from build123d import *

# Parameters (mm, degrees)
F0_R     = 9.75
F0_R_2   = 2.15
F1_DEPTH = 100


with BuildPart() as f1:
    # F0 (on Front) → F1 (new body)
    with BuildSketch(Plane.XZ):
        with Locations((6, 0)):
            Circle(F0_R)
        with Locations((3, -5.2)):
            Circle(F0_R_2, mode=Mode.SUBTRACT)
        with BuildLine():
            ThreePointArc((0.394847, -3.024334), (0.593975, -3.122706), (0.579462, -3.344334))
            ThreePointArc((0.579462, -3.344334), (-0.023044, -4.795398), (0.176673, -6.353832))
            ThreePointArc((0.176673, -6.353832), (0.105059, -6.594152), (-0.145019, -6.575618))
            ThreePointArc((-0.145019, -6.575618), (-1.795123, -4.498451), (-2.767969, -2.030449))
            ThreePointArc((-2.767969, -2.030449), (-2.65874, -1.804579), (-2.414779, -1.863154))
            ThreePointArc((-2.414779, -1.863154), (-1.164953, -2.818756), (0.394847, -3.024334))
        make_face(mode=Mode.SUBTRACT)
        with BuildLine():
            ThreePointArc((6.394847, -3.024334), (6.593975, -3.122706), (6.579462, -3.344334))
            ThreePointArc((6.579462, -3.344334), (6.359886, -3.672814), (6.184615, -4.026923))
            ThreePointArc((6.184615, -4.026923), (6, -4.15), (5.815385, -4.026923))
            ThreePointArc((5.815385, -4.026923), (5.640114, -3.672814), (5.420538, -3.344334))
            ThreePointArc((5.420538, -3.344334), (5.406025, -3.122706), (5.605153, -3.024334))
            ThreePointArc((5.605153, -3.024334), (6, -3.05), (6.394847, -3.024334))
        make_face(mode=Mode.SUBTRACT)
        with BuildLine():
            ThreePointArc((2.815385, -1.173077), (3, -1.05), (3.184615, -1.173077))
            ThreePointArc((3.184615, -1.173077), (3.359886, -1.527186), (3.579462, -1.855666))
            ThreePointArc((3.579462, -1.855666), (3.593975, -2.077294), (3.394847, -2.175666))
            ThreePointArc((3.394847, -2.175666), (3, -2.15), (2.605153, -2.175666))
            ThreePointArc((2.605153, -2.175666), (2.406025, -2.077294), (2.420538, -1.855666))
            ThreePointArc((2.420538, -1.855666), (2.640114, -1.527186), (2.815385, -1.173077))
        make_face(mode=Mode.SUBTRACT)
        with BuildLine():
            ThreePointArc((5.815385, -6.373077), (6, -6.25), (6.184615, -6.373077))
            ThreePointArc((6.184615, -6.373077), (7.139308, -7.616677), (8.585647, -8.221723))
            ThreePointArc((8.585647, -8.221723), (8.757847, -8.404014), (8.616624, -8.61123))
            ThreePointArc((8.616624, -8.61123), (6, -9), (3.383376, -8.61123))
            ThreePointArc((3.383376, -8.61123), (3.242153, -8.404014), (3.414353, -8.221723))
            ThreePointArc((3.414353, -8.221723), (4.860692, -7.616677), (5.815385, -6.373077))
        make_face(mode=Mode.SUBTRACT)
        with Locations((9, -5.2)):
            Circle(F0_R_2, mode=Mode.SUBTRACT)
        with BuildLine():
            ThreePointArc((8.815385, -1.173077), (9, -1.05), (9.184615, -1.173077))
            ThreePointArc((9.184615, -1.173077), (9.359886, -1.527186), (9.579462, -1.855666))
            ThreePointArc((9.579462, -1.855666), (9.593975, -2.077294), (9.394847, -2.175666))
            ThreePointArc((9.394847, -2.175666), (9, -2.15), (8.605153, -2.175666))
            ThreePointArc((8.605153, -2.175666), (8.406025, -2.077294), (8.420538, -1.855666))
            ThreePointArc((8.420538, -1.855666), (8.640114, -1.527186), (8.815385, -1.173077))
        make_face(mode=Mode.SUBTRACT)
        with BuildLine():
            ThreePointArc((11.420538, -3.344334), (11.406025, -3.122706), (11.605153, -3.024334))
            ThreePointArc((11.605153, -3.024334), (13.164953, -2.818756), (14.414779, -1.863154))
            ThreePointArc((14.414779, -1.863154), (14.65874, -1.804579), (14.767969, -2.030449))
            ThreePointArc((14.767969, -2.030449), (13.795123, -4.498451), (12.145019, -6.575618))
            ThreePointArc((12.145019, -6.575618), (11.894941, -6.594152), (11.823327, -6.353832))
            ThreePointArc((11.823327, -6.353832), (12.023044, -4.795398), (11.420538, -3.344334))
        make_face(mode=Mode.SUBTRACT)
        Circle(F0_R_2, mode=Mode.SUBTRACT)
        with BuildLine():
            ThreePointArc((0.579462, 3.344334), (0.593975, 3.122706), (0.394847, 3.024334))
            ThreePointArc((0.394847, 3.024334), (-1.164953, 2.818756), (-2.414779, 1.863154))
            ThreePointArc((-2.414779, 1.863154), (-2.65874, 1.804579), (-2.767969, 2.030449))
            ThreePointArc((-2.767969, 2.030449), (-1.795123, 4.498451), (-0.145019, 6.575618))
            ThreePointArc((-0.145019, 6.575618), (0.105059, 6.594152), (0.176673, 6.353832))
            ThreePointArc((0.176673, 6.353832), (-0.023044, 4.795398), (0.579462, 3.344334))
        make_face(mode=Mode.SUBTRACT)
        with BuildLine():
            ThreePointArc((3.184615, 1.173077), (3, 1.05), (2.815385, 1.173077))
            ThreePointArc((2.815385, 1.173077), (2.640114, 1.527186), (2.420538, 1.855666))
            ThreePointArc((2.420538, 1.855666), (2.406025, 2.077294), (2.605153, 2.175666))
            ThreePointArc((2.605153, 2.175666), (3, 2.15), (3.394847, 2.175666))
            ThreePointArc((3.394847, 2.175666), (3.593975, 2.077294), (3.579462, 1.855666))
            ThreePointArc((3.579462, 1.855666), (3.359886, 1.527186), (3.184615, 1.173077))
        make_face(mode=Mode.SUBTRACT)
        with Locations((3, 5.2)):
            Circle(F0_R_2, mode=Mode.SUBTRACT)
        with Locations((6, 0)):
            Circle(F0_R_2, mode=Mode.SUBTRACT)
        with BuildLine():
            ThreePointArc((9.184615, 1.173077), (9, 1.05), (8.815385, 1.173077))
            ThreePointArc((8.815385, 1.173077), (8.640114, 1.527186), (8.420538, 1.855666))
            ThreePointArc((8.420538, 1.855666), (8.406025, 2.077294), (8.605153, 2.175666))
            ThreePointArc((8.605153, 2.175666), (9, 2.15), (9.394847, 2.175666))
            ThreePointArc((9.394847, 2.175666), (9.593975, 2.077294), (9.579462, 1.855666))
            ThreePointArc((9.579462, 1.855666), (9.359886, 1.527186), (9.184615, 1.173077))
        make_face(mode=Mode.SUBTRACT)
        with BuildLine():
            ThreePointArc((5.605153, 3.024334), (5.406025, 3.122706), (5.420538, 3.344334))
            ThreePointArc((5.420538, 3.344334), (5.640114, 3.672814), (5.815385, 4.026923))
            ThreePointArc((5.815385, 4.026923), (6, 4.15), (6.184615, 4.026923))
            ThreePointArc((6.184615, 4.026923), (6.359886, 3.672814), (6.579462, 3.344334))
            ThreePointArc((6.579462, 3.344334), (6.593975, 3.122706), (6.394847, 3.024334))
            ThreePointArc((6.394847, 3.024334), (6, 3.05), (5.605153, 3.024334))
        make_face(mode=Mode.SUBTRACT)
        with Locations((12, 0)):
            Circle(F0_R_2, mode=Mode.SUBTRACT)
        with BuildLine():
            ThreePointArc((11.605153, 3.024334), (11.406025, 3.122706), (11.420538, 3.344334))
            ThreePointArc((11.420538, 3.344334), (12.023044, 4.795398), (11.823327, 6.353832))
            ThreePointArc((11.823327, 6.353832), (11.894941, 6.594152), (12.145019, 6.575618))
            ThreePointArc((12.145019, 6.575618), (13.795123, 4.498451), (14.767969, 2.030449))
            ThreePointArc((14.767969, 2.030449), (14.65874, 1.804579), (14.414779, 1.863154))
            ThreePointArc((14.414779, 1.863154), (13.164953, 2.818756), (11.605153, 3.024334))
        make_face(mode=Mode.SUBTRACT)
        with Locations((9, 5.2)):
            Circle(F0_R_2, mode=Mode.SUBTRACT)
        with BuildLine():
            ThreePointArc((6.184615, 6.373077), (6, 6.25), (5.815385, 6.373077))
            ThreePointArc((5.815385, 6.373077), (4.860692, 7.616677), (3.414353, 8.221723))
            ThreePointArc((3.414353, 8.221723), (3.242153, 8.404014), (3.383376, 8.61123))
            ThreePointArc((3.383376, 8.61123), (6, 9), (8.616624, 8.61123))
            ThreePointArc((8.616624, 8.61123), (8.757847, 8.404014), (8.585647, 8.221723))
            ThreePointArc((8.585647, 8.221723), (7.139308, 7.616677), (6.184615, 6.373077))
        make_face(mode=Mode.SUBTRACT)
    extrude(amount=F1_DEPTH)


solid = f1.part
Input: part model. Units: mm. Frame: model coordinates. Give positions to 0.01 mm unless a question says otherwise; leave off trailing zeros. Order: outer loops, then holes, each group sorted by start corner. A loop starts at its lowest first (then second) coordinate and runs counter-clockwise, first axis right, second up.
Q1. Section B-B on z = 5.2. Output: boundary loops of the cut face in (x, y), and give its area (3 significant figures).
Checked values:
outline: (-2.25, -100) - (-1.35, -100) - (-1.35, 0) - (-2.25, 0) - close; (-0.05, -100) - (0.85, -100) - (0.85, 0) - (-0.05, 0) - close; (5.15, -100) - (6.85, -100) - (6.85, 0) - (5.15, 0) - close; (11.15, -100) - (12.05, -100) - (12.05, 0) - (11.15, 0) - close; (13.35, -100) - (14.25, -100) - (14.25, 0) - (13.35, 0) - close
area: 530 mm2
Q2. Contact query for flat-ended pins moving along their axis: pin 1 Ø2.5 at (x, z) = (9, 5.2) entering from +Y; pin 2 Ø1.5 at (y, z) = (-39, 4) entering from -X; pin 3 Ø5 at (y, z) = (-75.5, -7) entering from +X; pin 4 Ø1 at (x, y) = (10.5, -48.5) entering from -Z. Output: stop coordinate, or through.
Checked values:
pin 1: passes through
pin 2: stops at x = -3.19
pin 3: stops at x = 14.65
pin 4: stops at z = -8.89
Q3. Section C-C on y = -69. State how many separate pieces and enclosed holes the cut face has, and give its area (3 significant figures).
Checked values:
separate pieces: 1
enclosed holes: 19
area: 150 mm2
Q4. Section A-A on z = 0. Output: boundary loops of the cut face in (x, y), and give its area (3 significant figures).
Checked values:
outline: (-3.75, -100) - (-2.15, -100) - (-2.15, 0) - (-3.75, 0) - close; (2.15, -100) - (3.85, -100) - (3.85, 0) - (2.15, 0) - close; (8.15, -100) - (9.85, -100) - (9.85, 0) - (8.15, 0) - close; (14.15, -100) - (15.75, -100) - (15.75, 0) - (14.15, 0) - close
area: 660 mm2
Q5. Ray query, probe 1 along Z at (x, y) = (3, -74); probe 2 along X at (y, z) = (-30, 5.75); probe 3 along Z at (x, y) = (8.25, -9.5). Return the intervals inside material, ascending.
Checked values:
probe 1: z = -9.28 to -7.35, -3.05 to -2.15, -1.05 to 1.05, 2.15 to 3.05, 7.35 to 9.28
probe 2: x = -1.87 to -0.92, 0 to 0.92, 5.08 to 6.92, 11.08 to 12, 12.92 to 13.87
probe 3: z = -9.49 to -8.71, -8.16 to -7.21, -3.19 to 3.19, 7.21 to 8.16, 8.71 to 9.49
Q6. Draft query along X for faces 1 (the flat face through (6.7, -100, 2.2)), 2 (the cylindrical face through (-2.15, -49.3, 0.09)). Return one class per face: +X half, -X half, draft (parallel to the pull), parting line (faces both ways), or undercut.
Checked values:
face 1: draft
face 2: undercut
